from build123d import *

# Parameters (mm, degrees)
ESTRUSIONE_ESTRUSIONE1_DEPTH = 3
ESTRUSIONE_ESTRUSIONE2_DEPTH = 6.6
SCHIZZO3_R                   = 1.75
TAGLIO_ESTRUSIONE1_DEPTH     = 20.442222095


with BuildPart() as part:
    # Schizzo1 → Estrusione-Estrusione1 (new, symmetric)
    with BuildSketch(Plane.XY):
        with BuildLine():
            Line((-13.8, 6), (13.8, 6))
            Line((13.8, 6), (13.8, -6))
            Line((13.8, -6), (5.979130372, -6))
            ThreePointArc((5.979130372, -6), (0, -0.5), (-5.979130372, -6))
            Line((-5.979130372, -6), (-13.8, -6))
            Line((-13.8, -6), (-13.8, 6))
        make_face()
    extrude(amount=ESTRUSIONE_ESTRUSIONE1_DEPTH, both=True)

    # Schizzo2 → Estrusione-Estrusione2 (add, symmetric)
    with BuildSketch(Plane.XY):
        with BuildLine():
            Line((13.8, 6), (-13.8, 6))
            Line((-13.8, 6), (-13.8, -6))
            Line((-13.8, -6), (-7.984359711, -6))
            ThreePointArc((-7.984359711, -6), (0, 1.5), (7.984359711, -6))
            Line((7.984359711, -6), (13.8, -6))
            Line((13.8, -6), (13.8, 6))
        make_face()
    extrude(amount=ESTRUSIONE_ESTRUSIONE2_DEPTH, both=True)

    # Schizzo3 → Taglio-Estrusione1 (cut, through all)
    with BuildSketch(Plane.XZ.offset(6)):
        with Locations((-10, 0)):
            Circle(SCHIZZO3_R)
        with Locations((10, 0)):
            Circle(SCHIZZO3_R)
    extrude(amount=-TAGLIO_ESTRUSIONE1_DEPTH, mode=Mode.SUBTRACT)


solid = part.part
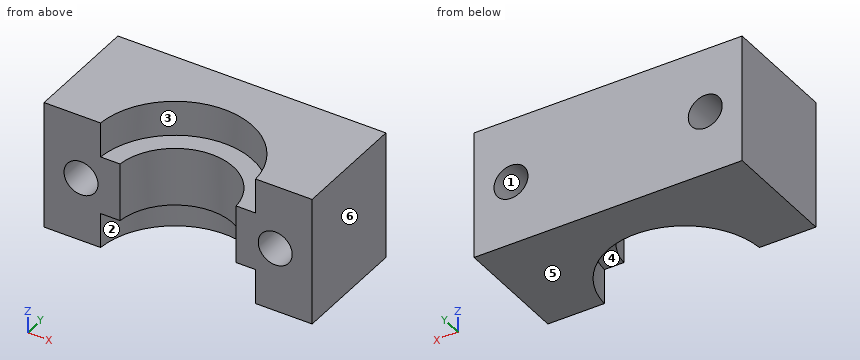
Build history of the part. All positions in model axes, mm. Face numbers are marked on the shaded views. A direction names the side the tool comes from. Round coordinates to 2 decimals unless told otherwise and drop trailing zeros. Write each loop counter-clockwise with the first axis right and the second up, starting at its lowest first coordinate (ties: lowest second). Pieces come first, ordered by that corner, then holes. Notation, with made-up numbers: (45.5, 65.25) -> (60.5, 65.25) arc R10 ccw to (60.5, 74.25) -> close; hole circle Ø10 at (2.25, 29). An arc over 180 degrees is marked (long way). Use one line per item in the form item = value.
Q1. Drill centre lines: L1, parallel to X at y = 2.5, z = -1.5; L2, parallel to Z at x = 10, y = 0.5; L3, parallel to Z at x = 5.75, y = -3.25. Where is each one in solid material? Low to high.
Conclusion:
L1 = -13.8 to -10.9, -9.1 to 9.1, 10.9 to 13.8
L2 = -6.6 to -1.75, 1.75 to 6.6
L3 = -3 to 3
Q2. Band-saw the part on D-D, the plane y = 0.5. Write the cut outline in (x, z).
Conclusion:
outline = (-13.8, -6.6) -> (-3.87, -6.6) -> (-3.87, -3) -> (3.87, -3) -> (3.87, -6.6) -> (13.8, -6.6) -> (13.8, 6.6) -> (3.87, 6.6) -> (3.87, 3) -> (-3.87, 3) -> (-3.87, 6.6) -> (-13.8, 6.6) -> close; hole circle Ø3.5 at (-10, 0); hole circle Ø3.5 at (10, 0)
Q3. Band-saw the part on C-C, the plane y = -3. Write the cut outline in (x, z), then the cut area to 3 significant figures.
Conclusion:
outline = (-13.8, -6.6) -> (-7.19, -6.6) -> (-7.19, -3) -> (-4.87, -3) -> (-4.87, 3) -> (-7.19, 3) -> (-7.19, 6.6) -> (-13.8, 6.6) -> close; (4.87, -3) -> (7.19, -3) -> (7.19, -6.6) -> (13.8, -6.6) -> (13.8, 6.6) -> (7.19, 6.6) -> (7.19, 3) -> (4.87, 3) -> close; hole circle Ø3.5 at (-10, 0); hole circle Ø3.5 at (10, 0)
area = 183 mm²
Q4. Two-plate mould, pull along X, no slides. Class the marked faces 4, 5 and 6: released by +X, released by -X, zero draft, split by the parting line, or undercut.
Conclusion:
face_4 = undercut
face_5 = zero draft
face_6 = released by +X
Q5. Drop flat-ended pins along their axis: P1, Ø1.5, axis at x = 4.5, y = -1.5, coming from the -Z side; P2, Ø3.5, axis at x = -3.5, y = -2.5, coming from the +Z side. Give the stop position or say it passes through.
Conclusion:
P1 = -3
P2 = 3
Q6. Band-saw the part on A-A, the plane z = 0. Write the cut outline in (x, y), then the cut area to 3 significant figures.
Conclusion:
outline = (-13.8, -6) -> (-11.75, -6) -> (-11.75, 6) -> (-13.8, 6) -> close; (-8.25, -6) -> (-5.98, -6) arc R6 cw to (5.98, -6) -> (8.25, -6) -> (8.25, 6) -> (-8.25, 6) -> close; (11.75, -6) -> (13.8, -6) -> (13.8, 6) -> (11.75, 6) -> close
area = 197 mm²
Q7. Tool access for the marked faces 1, 2 and 3: list every direction of +Z, -Z, +X, -X, +Y, -Y with a clear straight run to the whole face (end or side of a thin tool).
Conclusion:
face_1 = +Y, -Y
face_2 = -Z, -Y
face_3 = +Z, -Y
Q8. Band-saw the part on B-B, the plane x = -10. Write the cut outline in (y, z), then the cut area to 3 significant figures.
Conclusion:
outline = (-6, -6.6) -> (6, -6.6) -> (6, -1.75) -> (-6, -1.75) -> close; (-6, 1.75) -> (6, 1.75) -> (6, 6.6) -> (-6, 6.6) -> close
area = 116 mm²
